Could you check a few things on this model? Use its own coordinates, in mm. A direction names the side the tool comes from. Round coordinates to 2 decimals unless told otherwise and drop trailing zeros. Loops run counter-clockwise (first coordinate to the right, second up) from the corner with the lowest first, then second, coordinate; pieces in that order, holes last. Notation, with made-up numbers: (14, 31) -> (61, 31) arc R26 cw to (61, 53) -> close; hole circle Ø5 at (56.5, -17). An arc over 180 degrees is marked (long way). Write each question's results on one line, items separated by ' | '. Start each with the question number.
1) Which directions (+Z, -Z, +X, -X, +Y, -Y) give clear straight access to the entire face, cutting with the end or side of a thin tool? Please do faces 5 (the flat face through (-10, 0, 0)), 6 (the flat face through (27.816, 25, 2)), 7 (the flat face through (32.116, -25, 2)), 8 (the flat face through (-71, -5.75, 2)), 9 (the flat face through (30, -4.15, 2)).
2) Imagine slicing it at B-B, the plane z = 2.65. Give the number of separate pieces and of enclosed holes in the cut face, plus the area to 3 significant figures.
3) If I drill on probe 1 along Y at (x, z) = (-39, 2.7); probe 2 along Y at (x, z) = (-28, 3.85); probe 3 along X at (y, z) = (-13.5, 1.9), over which ranges is the centre line in solid material (lowest first)?
4) Imagine slicing it at A-A, the plane y = 0. List the corners of the cut face in (x, z) for me, plus the area to 3 significant figures.
5) For P1, Ø2, axis at x = -67.5, z = 2.5, coming from the +Y side; P2, Ø2, axis at x = -29.04, y = 5.75, coming from the -Z side; P3, Ø1.5, axis at x = -51, z = 1, coming from the +Y side; P4, Ø1, axis at x = -49, z = 1, coming from the +Y side, each with a flat end and sliding along its axis, tell me the tip position at first contact or that it passes through.
6) We'd pull the mould along X, two halves only. Please class faces 1 (the cylindrical face through (-42, 0, 2)), 2 (the flat face through (-1, -27.15, 2)), 3 (the flat face through (36.001, 0, 2)), 4 (the cylindrical face through (-38.327, 12.554, 1.972)): pulls with the +X half, pulls with the -X half, needs draft (parallel to the pull), parting line crosses it, or undercut.
from build123d import *

# Parameters (mm, degrees)
SKETCH_1_R      = 1.5
SKETCH_1_R_2    = 3
SKETCH_1_R_3    = 1.25
SKETCH_1_R_4    = 2
SKETCH_1_W      = 4.3
SKETCH_1_H      = 8.3
EXTRUDE_1_DEPTH = 4


with BuildPart() as part:
    # 草图1 → 凸台-拉伸1 (new body)
    with BuildSketch(Plane.XY):
        with BuildLine():
            Line((32.115707856, 27.15), (32.115707856, 22.85))
            Line((32.115707856, 22.85), (27.815707856, 22.85))
            Line((27.815707856, 22.85), (27.815707856, 27.15))
            Line((27.815707856, 27.15), (-29.075, 27.15))
            Line((-29.075, 27.15), (-38.998995168, 22.002009663))
            ThreePointArc((-38.998995168, 22.002009663), (-52.370174504, 17.472835843), (-60.236366221, 5.75))
            Line((-60.236366221, 5.75), (-80.958287312, 5.75))
            Line((-80.958287312, 5.75), (-80.958287312, -5.75))
            Line((-80.958287312, -5.75), (-60.236366221, -5.75))
            ThreePointArc((-60.236366221, -5.75), (-52.370174504, -17.472835843), (-38.998995168, -22.002009663))
            Line((-38.998995168, -22.002009663), (-29.075, -27.15))
            Line((-29.075, -27.15), (27.815707856, -27.15))
            Line((27.815707856, -27.15), (27.815707856, -22.85))
            Line((27.815707856, -22.85), (32.115707856, -22.85))
            Line((32.115707856, -22.85), (32.115707856, -27.15))
            Line((32.115707856, -27.15), (36.001004832, -27.15))
            Line((36.001004832, -27.15), (36.001004832, 27.15))
            Line((36.001004832, 27.15), (32.115707856, 27.15))
        make_face()
        with Locations((30.001004832, 13.5)):
            Circle(SKETCH_1_R, mode=Mode.SUBTRACT)
        with Locations(Location((30.001004832, -13.5, 0), (0, 0, 180))):
            Circle(SKETCH_1_R, mode=Mode.SUBTRACT)
        with Locations((-38.998995168, 0)):
            Circle(SKETCH_1_R_2, mode=Mode.SUBTRACT)
        with Locations((-38.998995168, -11.5)):
            Circle(SKETCH_1_R_3, mode=Mode.SUBTRACT)
        with Locations((-48.958287312, -5.75)):
            Circle(SKETCH_1_R_3, mode=Mode.SUBTRACT)
        with Locations((-48.958287312, 5.75)):
            Circle(SKETCH_1_R_3, mode=Mode.SUBTRACT)
        with Locations((-38.998995168, 11.5)):
            Circle(SKETCH_1_R_3, mode=Mode.SUBTRACT)
        with Locations((-29.039703025, 5.75)):
            Circle(SKETCH_1_R_3, mode=Mode.SUBTRACT)
        with Locations((-29.039703025, -5.75)):
            Circle(SKETCH_1_R_3, mode=Mode.SUBTRACT)
        with Locations((-4.075, -22.15)):
            Circle(SKETCH_1_R_4, mode=Mode.SUBTRACT)
        with Locations((-4.075, 22.15)):
            Circle(SKETCH_1_R_4, mode=Mode.SUBTRACT)
        with Locations((-76.958287312, 0)):
            Circle(SKETCH_1_R_4, mode=Mode.SUBTRACT)
        with Locations((30.001004832, 0)):
            Rectangle(SKETCH_1_W, SKETCH_1_H, mode=Mode.SUBTRACT)
    extrude(amount=EXTRUDE_1_DEPTH)


solid = part.part
Checked values:
1) face 5: -Z, +X, -X, +Y, -Y | face 6: +Z, -Z, +Y | face 7: +Z, -Z, -Y | face 8: +Z, -Z, -X, -Y | face 9: +Z, -Z
2) separate pieces: 1 | enclosed holes: 13 | area: 4,830 mm^2
3) probe 1: -22 to -12.75, -10.25 to -3, 3 to 10.25, 12.75 to 22 | probe 2: -27.15 to -6.44, -5.06 to 5.06, 6.44 to 27.15 | probe 3: -56.37 to 28.5, 31.5 to 36
4) outline: (-80.96, 0) -> (-78.96, 0) -> (-78.96, 4) -> (-80.96, 4) -> close; (-74.96, 0) -> (-42, 0) -> (-42, 4) -> (-74.96, 4) -> close; (-36, 0) -> (27.85, 0) -> (27.85, 4) -> (-36, 4) -> close; (32.15, 0) -> (36, 0) -> (36, 4) -> (32.15, 4) -> close | area: 411 mm^2
5) P1: y = 5.75 | P2: through | P3: y = 18.91 | P4: y = 19.84
6) face 1: undercut | face 2: needs draft | face 3: pulls with the +X half | face 4: undercut
